```python
from build123d import *

# Parameters (mm, degrees)
SKETCH1_R           = 50
BOSS_EXTRUDE1_DEPTH = 15
CUT_EXTRUDE1_START  = -10
CUT_EXTRUDE1_DEPTH  = 10
SKETCH3_R           = 20
BOSS_EXTRUDE2_DEPTH = 25


with BuildPart() as part:
    # Sketch1 → Boss-Extrude1 (new body)
    with BuildSketch(Plane(origin=(0, 0, 0), x_dir=(1, 0, 0), z_dir=(0, 1, 0))):
        with Locations(Location((0, 0, 0), (0, 0, 270))):
            Circle(SKETCH1_R)
    extrude(amount=BOSS_EXTRUDE1_DEPTH)

    # Sketch2 → Cut-Extrude1 (cut)
    with BuildSketch(Plane(origin=(0, 15, 0), x_dir=(1, 0, 0), z_dir=(0, 1, 0)).offset(CUT_EXTRUDE1_START)):
        with BuildLine():
            Line((-5, 49.749371855), (-5, -49.749371855))
            ThreePointArc((-5, -49.749371855), (0, -50), (5, -49.749371855))
            Line((5, -49.749371855), (5, 49.749371855))
            ThreePointArc((5, 49.749371855), (0, 50), (-5, 49.749371855))
        make_face()
    extrude(amount=CUT_EXTRUDE1_DEPTH, mode=Mode.SUBTRACT)

    # Sketch3 → Boss-Extrude2 (add)
    with BuildSketch(Plane.XZ):
        with Locations(Location((0, 0, 0), (0, 0, 90))):
            Circle(SKETCH3_R)
        with BuildLine():
            Line((3, 18.696938457), (3, 14.696938457))
            ThreePointArc((3, 14.696938457), (11.618950039, 9.486832981), (15, 0))
            ThreePointArc((15, 0), (-9.486832981, -11.618950039), (-3, 14.696938457))
            Line((-3, 14.696938457), (-3, 18.696938457))
            Line((-3, 18.696938457), (3, 18.696938457))
        make_face(mode=Mode.SUBTRACT)
    extrude(amount=BOSS_EXTRUDE2_DEPTH)


solid = part.part
```
Geometry check sheet. Reference: the model listing, model coordinates, mm. A direction names the side the tool comes from. Give positions to 0.01 mm unless a question says otherwise; leave off trailing zeros. Order: outer loops, then holes, each group sorted by start corner. A loop starts at its lowest first (then second) coordinate and runs counter-clockwise, first axis right, second up.
1. Gauge pin test, flat ends, axial feed: pin 1 Ø4 at (y, z) = (-8, 12.5) entering from +X; pin 2 Ø2 at (x, z) = (4.5, -12.5) entering from -Y; pin 3 Ø10 at (y, z) = (-17, -11.5) entering from -X; pin 4 Ø24 at (x, z) = (6.5, -4) entering from -Y. Record the tip position at first contact, or that the pin passes through.
2. Release check for a two-part mould opening along Z. For faces 4 (the face through (-5, 10, -1)), 5 (the face through (19.524, -12.325, -4.336)), 6 (the face through (-3, -12, 17)) record: pulls with the +Z half, pulls with the -Z half, needs draft (parallel to the pull), parting line crosses it, or undercut.
3. Section check C-C, the plane y = -5. Enter the section's corners in (x, z).
4. Section check B-B, the plane x = 0. Enter the section's corners in (y, z), and give its area (3 significant figures).
5. Section check A-A, the plane z = -40. Enter the section's corners in (x, y).
6. Section check D-D, the plane y = 3.5. Enter the section's corners in (x, z), and give its area (3 significant figures).
7. Access from +Z, -Z, +X, -X, +Y, -Y to the whole of each face (thin tool, end or side, straight path). Record for faces 1 (the face through (15.02, 7.4, 47.69)), 2 (the face through (0, -12, 18.697)), 3 (the face through (0, 5, -1)).
8. Thickness scan on L1, parallel to X at y = -14.5, z = 0; L2, parallel to Y at x = 38.5, z = 27.5; L3, parallel to X at y = 13.5, z = -23.5. Record the ranges inside material, lowest first.
Values follow:
1. pin 1: stops at x = 17.02
1. pin 2: stops at y = 0
1. pin 3: stops at x = -18.91
1. pin 4: stops at y = -25
2. face 4: needs draft
2. face 5: parting line crosses it
2. face 6: undercut
3. outline: circle Ø40 at (0, 0); hole (-3, 14.7) arc R15 ccw (long way) to (3, 14.7) - (3, 18.7) - (-3, 18.7) - close
4. outline: (-25, -20) - (0, -20) - (0, -50) - (5, -50) - (5, 50) - (0, 50) - (0, 20) - (-25, 20) - (-25, 18.7) - (0, 18.7) - (0, -15) - (-25, -15) - close
4. area: 658 mm2
5. outline: (-30, 0) - (30, 0) - (30, 15) - (5, 15) - (5, 5) - (-5, 5) - (-5, 15) - (-30, 15) - close
6. outline: circle Ø100 at (0, 0)
6. area: 7,850 mm2
7. face 1: +Y, -Y
7. face 2: -Y
7. face 3: +Z, -Z, +Y
8. L1: x = -20 to -15, 15 to 20
8. L2: y = 0 to 15
8. L3: x = -44.13 to -5, 5 to 44.13
